Source: CAD feature listing. Evaluate the final solid. Frame: model axes, mm. A direction names the side the tool comes from. Round coordinates to 2 decimals unless told otherwise and drop trailing zeros. Order: outer loops, then holes, each group sorted by start corner. A loop starts at its lowest first (then second) coordinate and runs counter-clockwise, first axis right, second up. Notation, with made-up numbers: (71.25, -2.75) -> (101.25, -2.75) arc R10 ccw to (101.25, 13.25) -> close; hole circle Ø11 at (6, -32). An arc over 180 degrees is marked (long way). Answer as CSV lines item,"result". Start each with the question number.
(1) Section query A-A (z = 13.5). Output: boundary loops of the cut face in (x, y) (1 decimal), plus the area to 3 significant figures.
(2) Section query C-C (y = -13). Output: boundary loops of the cut face in (x, z) (3 decimals).
(3) Pull-direction query (X, two-part tool) for faces 3 (the cylindrical face through (32.56, -33.17, 6.26)), 4 (the flat face through (-34.925, -20, 13)), 5 (the flat face through (34.925, -20, 13)); classes: +X half, -X half, draft (parallel to the pull), parting line (faces both ways), or undercut.
(4) Line query: line 1 along X through (y, z) = (-33, 12.5) (3 decimals); line 2 along Y through (x, z) = (-25.4, 11.25); line 3 along Y through (x, z) = (-29, 7). Output: solid intervals per line, ascending. Write a range as from..to.
(5) Set-up query: faces 1 (the cylindrical face through (32.56, -7.77, 6.26)), 2 (the flat face through (31, -20, 0)). Return all of +Z, -Z, +X, -X, +Y, -Y with unobstructed straight access to the full face (end or side cutting, diameter ignored); none if empty.
(6) Section query D-D (z = 6.5). Output: boundary loops of the cut face in (x, y) (1 decimal), plus the area to 3 significant figures.
(7) Section query B-B (x = 25.4). Output: boundary loops of the cut face in (y, z), plus the area to 3 significant figures.
```python
from build123d import *

# Parameters (mm, degrees)
BOSS_EXTRUDE2_DEPTH                                = 39.878
FILLET1_R                                          = 0.635
CSK_FOR_10_FLAT_HEAD_MACHINE_SCREW_100_D           = 5.1054
CSK_FOR_10_FLAT_HEAD_MACHINE_SCREW_100_CSINK_D     = 9.779
CSK_FOR_10_FLAT_HEAD_MACHINE_SCREW_100_CSINK_ANGLE = 82
F_10_0_1935_DIAMETER_HOLE2_AT_2_COUNT              = 2
F_10_0_1935_DIAMETER_HOLE2_AT_2_PITCH              = 25.4


with BuildPart() as part:
    # Sketch5 → Boss-Extrude2 (new body)
    with BuildSketch(Plane(origin=(0, 0, 0), x_dir=(1, 0, 0), z_dir=(0, 1, 0))):
        with BuildLine():
            Line((-34.925, 0), (-34.925, -25.4))
            Line((-34.925, -25.4), (34.925, -25.4))
            Line((34.925, -25.4), (34.925, 0))
            Line((34.925, 0), (19.05, 0))
            ThreePointArc((19.05, 0), (0, -19.05), (-19.05, 0))
            Line((-19.05, 0), (-34.925, 0))
        make_face()
    extrude(amount=-BOSS_EXTRUDE2_DEPTH)

    # Fillet1
    fillet1_edges = [part.edges().sort_by_distance(p)[0] for p in [
        (-19.05, -19.939, 0),
        (19.05, -19.939, 0),
    ]]
    fillet(fillet1_edges, radius=FILLET1_R)

    # CSK for #10 Flat Head Machine Screw (100)1 (through all)
    with Locations(Plane(origin=(0, 0, 0), x_dir=(-1, 0, 0), z_dir=(0, 0, -1))):
        with Locations((-25.4, -19.939)):
            csk_for_10_flat_head_machine_screw_100 = CounterSinkHole(CSK_FOR_10_FLAT_HEAD_MACHINE_SCREW_100_D / 2, CSK_FOR_10_FLAT_HEAD_MACHINE_SCREW_100_CSINK_D / 2, counter_sink_angle=CSK_FOR_10_FLAT_HEAD_MACHINE_SCREW_100_CSINK_ANGLE)

    # Sketch12 → #10 (0.1935) Diameter Hole2 (revolve, cut)
    with BuildSketch(Plane(origin=(30.1625, -7.239, 0), x_dir=(0, 1, 0), z_dir=(1, 0, 0))):
        Polygon((0, 0), (0, 14.176584928), (2.45745, 12.7), (2.45745, 0), align=None)
    f_10_0_1935_diameter_hole2 = revolve(axis=Axis((30.1625, -7.239, -6.35), (0, 0, 1)), mode=Mode.SUBTRACT)

    # #10 (0.1935) Diameter Hole2 at 2: #10 (0.1935) Diameter Hole2 ×2
    with Locations(*[(0, -i * F_10_0_1935_DIAMETER_HOLE2_AT_2_PITCH, 0) for i in range(1, F_10_0_1935_DIAMETER_HOLE2_AT_2_COUNT)]):
        add(f_10_0_1935_diameter_hole2, mode=Mode.SUBTRACT)

    # Mirror1: #10 (0.1935) Diameter Hole2, CSK for #10 Flat Head Machine Screw (100)1 across plane
    add(f_10_0_1935_diameter_hole2.mirror(Plane(origin=(0, 0, 0), x_dir=(0, 0, 1), z_dir=(1, 0, 0))), mode=Mode.SUBTRACT)
    add(csk_for_10_flat_head_machine_screw_100.mirror(Plane(origin=(0, 0, 0), x_dir=(0, 0, 1), z_dir=(1, 0, 0))), mode=Mode.SUBTRACT)

    # Mirror1 copy 1 sketch → Mirror1 copy 1 (revolve, cut)
    with BuildSketch(Plane(origin=(-30.1625, -32.639, 0), x_dir=(0, 1, 0), z_dir=(-1, 0, 0))):
        Polygon((0, 0), (0, -14.176584928), (2.45745, -12.7), (2.45745, 0), align=None)
    revolve(axis=Axis((-30.1625, -32.639, -6.35), (0, 0, -1)), mode=Mode.SUBTRACT)


solid = part.part
```
Answer block:
1,outline,"(-34.9, -39.9) -> (-13.4, -39.9) -> (-13.4, 0) -> (-34.9, 0) -> close; (13.4, -39.9) -> (34.9, -39.9) -> (34.9, 0) -> (13.4, 0) -> close; hole circle Ø2.3 at (-30.2, -32.6); hole circle Ø2.3 at (-30.2, -7.2); hole circle Ø5.1 at (-25.4, -19.9); hole circle Ø5.1 at (25.4, -19.9); hole circle Ø2.3 at (30.2, -32.6); hole circle Ø2.3 at (30.2, -7.2)"
1,area,"1,660 mm2"
2,outline,"(-34.925, 0) -> (-19.675, 0) arc R0.635 ccw to (-19.04, 0.615) arc R19.05 cw to (19.04, 0.615) arc R0.635 ccw to (19.675, 0) -> (34.925, 0) -> (34.925, 25.4) -> (-34.925, 25.4) -> close"
3,face 3,"undercut"
3,face 4,"-X half"
3,face 5,"+X half"
4,line 1,"-34.925..-32.593, -27.732..-14.375, 14.375..27.732, 32.593..34.925"
4,line 2,"-39.88..-22.49, -17.39..0"
4,line 3,"-39.88..-34.8, -30.47..-9.4, -5.07..0"
5,face 1,"-Z"
5,face 2,"-Z, +X, -X, +Y, -Y"
6,outline,"(-34.9, -39.9) -> (-17.9, -39.9) -> (-17.9, 0) -> (-34.9, 0) -> close; (17.9, -39.9) -> (34.9, -39.9) -> (34.9, 0) -> (17.9, 0) -> close; hole circle Ø4.9 at (-30.2, -32.6); hole circle Ø4.9 at (-30.2, -7.2); hole circle Ø5.1 at (-25.4, -19.9); hole circle Ø5.1 at (25.4, -19.9); hole circle Ø4.9 at (30.2, -32.6); hole circle Ø4.9 at (30.2, -7.2)"
6,area,"1,240 mm2"
7,outline,"(-39.88, 0) -> (-24.83, 0) -> (-22.49, 2.69) -> (-22.49, 25.4) -> (-39.88, 25.4) -> close; (-17.39, 2.69) -> (-15.05, 0) -> (0, 0) -> (0, 25.4) -> (-17.39, 25.4) -> close"
7,area,"877 mm2"
